Can you work these out from the drawing? Everything is in mm from the part's minimum corner. Coordinates: 2 decimals unless noted, no trailing zeros. Order: outer loops, then holes, each group sorted by start corner. A loop starts at its lowest first (then second) coordinate and runs counter-clockwise, first axis right, second up. Notation, with made-up numbers: (-29, 8) - (4, 8) arc R13 cw to (4, 21) - close; hole circle Ø2 at (61.5, -37). An arc over 180 degrees is marked (long way). One line per item, written item: value.
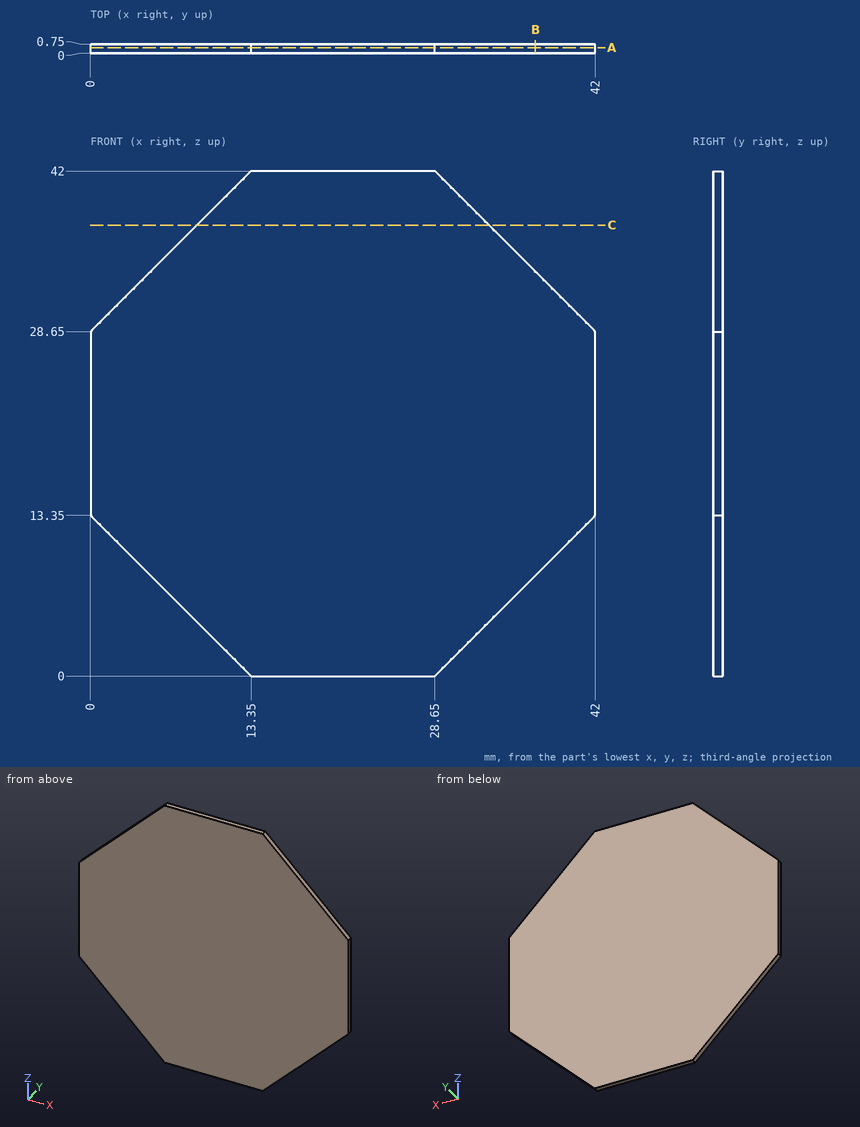
Item 1: If I drill on probe 1 along X at (y, z) = (0.25, 9.5); probe 2 along X at (y, z) = (0.4, 5.5); probe 3 along Z at (x, y) = (35.5, 0.4), over which ranges is the centre line in solid material (lowest first)?
Conclusion:
probe 1: 3.85 to 38.15
probe 2: 7.85 to 34.15
probe 3: 6.85 to 35.15
Item 2: I want a section at C-C on z = 37.5. Please give me the cut outline in (x, y), then the cut area to 3 significant figures.
Conclusion:
outline: (8.85, 0) - (33.15, 0) - (33.15, 0.75) - (8.85, 0.75) - close
area: 18.2 mm²
Item 3: I'm going to push a flat-ended pin straight in: pin 1 Ø1 at (x, z) = (37.5, 35) entering from +Y. Where does the tip first touch, or does it pass through?
Conclusion:
pin 1: through
Item 4: I want a section at B-B on x = 37. Please give me the cut outline in (y, z), then the cut area to 3 significant figures.
Conclusion:
outline: (0, 8.35) - (0.75, 8.35) - (0.75, 33.65) - (0, 33.65) - close
area: 19.0 mm²
Item 5: I want a section at A-A on y = 0.45. Please give me the cut outline in (x, z), then the cut area to 3 significant figures.
Conclusion:
outline: (0, 13.35) - (13.35, 0) - (28.65, 0) - (42, 13.35) - (42, 28.65) - (28.65, 42) - (13.35, 42) - (0, 28.65) - close
area: 1,410 mm²
